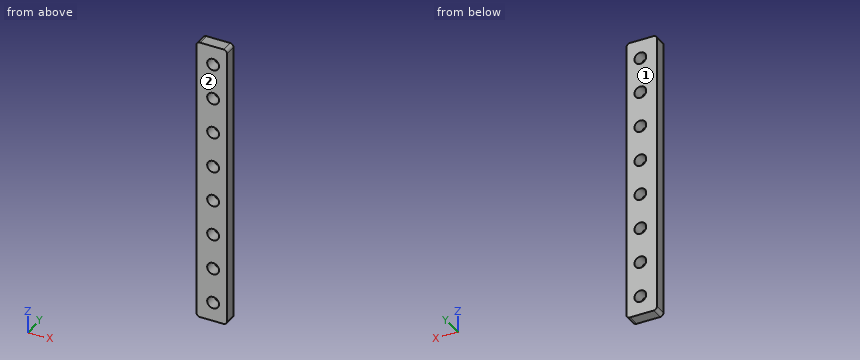
from build123d import *

# Parameters (mm, degrees)
SKETCH1_W            = 22
SKETCH1_H            = 205
BOSS_EXTRUDE1_DEPTH  = 8.7
M8_CLEARANCE_HOLE1_D = 8.5
LPATTERN1_COUNT      = 8
LPATTERN1_PITCH      = 25.4
FILLET1_R            = 2.5


with BuildPart() as part:
    # Sketch1 → Boss-Extrude1 (new body)
    with BuildSketch(Plane(origin=(0, 0, 0), x_dir=(1, 0, 0), z_dir=(0, 1, 0))):
        with Locations((-1, 0)):
            Rectangle(SKETCH1_W, SKETCH1_H)
    extrude(amount=BOSS_EXTRUDE1_DEPTH)

    # M8 Clearance Hole1 (through all)
    with Locations(Plane.XZ):
        with Locations((0, 88.9)):
            m8_clearance_hole1 = Hole(M8_CLEARANCE_HOLE1_D / 2)

    # LPattern1: M8 Clearance Hole1 ×8
    with Locations(*[(0, 0, -i * LPATTERN1_PITCH) for i in range(1, LPATTERN1_COUNT)]):
        add(m8_clearance_hole1, mode=Mode.SUBTRACT)

    # Fillet1
    fillet1_edges = [part.edges().sort_by_distance(p)[0] for p in [
        (10, 4.35, 102.5),
        (-12, 4.35, 102.5),
        (-12, 4.35, -102.5),
        (10, 4.35, -102.5),
    ]]
    fillet(fillet1_edges, radius=FILLET1_R)


solid = part.part
Input: part model. Units: mm. Frame: model coordinates. Face numbers are marked on the shaded views. Give positions to 0.01 mm unless a question says otherwise; leave off trailing zeros. Loops run counter-clockwise (first coordinate to the right, second up) from the corner with the lowest first, then second, coordinate; pieces in that order, holes last. Notation, with made-up numbers: (67, 58.25) -> (122, 58.25) arc R21 ccw to (122, 83.25) -> close; hole circle Ø6 at (65, -36). An arc over 180 degrees is marked (long way). Answer as a JSON object with one key per item and string values. Group by question number.
Item 1: Pull-direction query (Y, two-part tool) for the marked faces 1 and 2; classes: released by +Y, released by -Y, zero draft, split by the parting line, or undercut.
Item 2: Line query: probe 1 along X at (y, z) = (5.25, -92); probe 2 along X at (y, z) = (7, 36.5); probe 3 along Z at (x, y) = (-10.75, 1). Output: solid intervals per line, ascending.
Item 3: Pin query (flat end, axial travel): P1, Ø5, axis at x = 0, z = -63.5, coming from the -Y side. Return the tip coordinate at first contact, or that it passes through.
Item 4: Cut plane A-A, the plane z = -63.5. Return the cut outline in (x, y).
Item 5: Cut plane B-B, the plane y = 6.25. State how many separate pieces and enclosed holes the cut face has, and give its area (3 significant figures).
Checks:
{
 "1": {"face 1": "released by +Y", "face 2": "released by -Y"},
 "2": {"probe 1": "x = -12 to -2.91, 2.91 to 10", "probe 2": "x = -12 to -3.94, 3.94 to 10", "probe 3": "z = -102.17 to 102.17"},
 "3": {"P1": "passes through"},
 "4": {"outline": "(-12, 0) -> (-4.25, 0) -> (-4.25, 8.7) -> (-12, 8.7) -> close; (4.25, 0) -> (10, 0) -> (10, 8.7) -> (4.25, 8.7) -> close"},
 "5": {"separate pieces": "1", "enclosed holes": "8", "area": "4,050 mm²"}
}
